Verification items for the finished model (mm, model axes). A direction names the side the tool comes from. Give positions to 0.01 mm unless a question says otherwise; leave off trailing zeros. Write each loop counter-clockwise with the first axis right and the second up, starting at its lowest first coordinate (ties: lowest second). Pieces come first, ordered by that corner, then holes. Notation, with made-up numbers: (83, -5) -> (89, -5) arc R26 ccw to (89, 14) -> close; hole circle Ø8 at (33.5, -25.5). An arc over 180 degrees is marked (long way). Use CSV: the item, a comma, the result in double quotes. Start each with the question number.
```python
from build123d import *

# Parameters (mm, degrees)
SKETCH1_R           = 1.5
BOSS_EXTRUDE1_DEPTH = 5
SKETCH2_R           = 6.375
CUT_EXTRUDE1_DEPTH  = 10
SKETCH3_W           = 16
SKETCH3_H           = 24.75
CUT_EXTRUDE2_DEPTH  = 10
FILLET1_R           = 2


with BuildPart() as part:
    # Sketch1 → Boss-Extrude1 (new body)
    with BuildSketch(Plane(origin=(0, 0, 0), x_dir=(1, 0, 0), z_dir=(0, 1, 0))):
        Polygon((5, -14), (19, -14), (19, -9), (24, -9), (24, 48.5), (19, 48.5), (19, 53.5), (5, 53.5), (5, 48.5), (0, 48.5), (0, -9), (5, -9), align=None)
        with Locations(Location((12, 51, 0), (0, 0, 270))):
            Circle(SKETCH1_R, mode=Mode.SUBTRACT)
        with Locations(Location((12, -11.5, 0), (0, 0, 90))):
            Circle(SKETCH1_R, mode=Mode.SUBTRACT)
    extrude(amount=BOSS_EXTRUDE1_DEPTH)

    # Sketch2 → Cut-Extrude1 (cut)
    with BuildSketch(Plane(origin=(0, 5, 0), x_dir=(1, 0, 0), z_dir=(0, 1, 0))):
        with Locations(Location((12, 29.26, 0), (0, 0, 270))):
            Circle(SKETCH2_R)
    extrude(amount=-CUT_EXTRUDE1_DEPTH, mode=Mode.SUBTRACT)

    # Sketch3 → Cut-Extrude2 (cut)
    with BuildSketch(Plane(origin=(0, 5, 0), x_dir=(1, 0, 0), z_dir=(0, 1, 0))):
        with Locations((12, 7.375)):
            Rectangle(SKETCH3_W, SKETCH3_H)
    extrude(amount=-CUT_EXTRUDE2_DEPTH, mode=Mode.SUBTRACT)

    # Fillet1
    fillet1_edges = [part.edges().sort_by_distance(p)[0] for p in [
        (20, 2.5, 5),
        (4, 2.5, 5),
        (4, 2.5, -19.75),
        (20, 2.5, -19.75),
    ]]
    fillet(fillet1_edges, radius=FILLET1_R)


solid = part.part
```
(1) Set-up check for faces 4 (the face through (2, 2, 9)), 5 (the face through (12, 3, 5)), 6 (the face through (19, 2, 12)): record each of +Z, -Z, +X, -X, +Y, -Y from which the full face is reachable in a straight line by a thin tool's end or side.
(2) Go/stop test with flat-tipped pins: pin 1 (2.5 mm diameter, centred on x = 1.5, y = 1.5, fed in from +Z); pin 2 (1.5 mm diameter, centred on x = 2.5, y = 3, fed in from -Z); pin 3 (1.5 mm diameter, centred on y = 3, z = 10.5, fed in from +X). Record where each tip stops, or that it passes through.
(3) Section check C-C on y = 2.75. Record the cut outline in (x, z) (3 decimals), then the cut area to 3 significant figures.
(4) Section check B-B on x = 12. Record the cut outline in (y, z) (3 decimals), then the cut area to 3 significant figures.
(5) Draft check along Z on faces 1 (the face through (3, 2, -48.5)), 2 (the face through (20, 3, -7)), 3 (the face through (12, 5, -20)). Enter one of: released by +Z, released by -Z, zero draft, split by the parting line, or undercut.
(6) Section check D-D on z = -29.26. Record the cut outline in (x, y) (3 decimals), then the cut area to 4 significant figures.
(7) Section check A-A on z = -51. Record the cut outline in (x, y), then the cut area to 3 significant figures.
(8) Thickness scan on line 1 (X direction, y = 1.3, z = 11.5); line 2 (Z direction, x = 6.75, y = 2.45); line 3 (Z direction, x = 9, y = 1.45) (3 decimals). Record the ranges inside material, lowest first. Write a range as from..to.
Data:
1,face 4,"+Z, -X, +Y, -Y"
1,face 5,"+Y, -Y"
1,face 6,"+Z, +X, +Y, -Y"
2,pin 1,"stops at z = 9"
2,pin 2,"stops at z = -48.5"
2,pin 3,"stops at x = 19"
3,outline,"(0, -48.5) -> (5, -48.5) -> (5, -53.5) -> (19, -53.5) -> (19, -48.5) -> (24, -48.5) -> (24, 9) -> (19, 9) -> (19, 14) -> (5, 14) -> (5, 9) -> (0, 9) -> close; hole (4, -17.75) arc R2 ccw to (6, -19.75) -> (18, -19.75) arc R2 ccw to (20, -17.75) -> (20, 3) arc R2 ccw to (18, 5) -> (6, 5) arc R2 ccw to (4, 3) -> close; hole circle Ø12.75 at (12, -29.26); hole circle Ø3 at (12, -51); hole circle Ø3 at (12, 11.5)"
3,area,"986 mm2"
4,outline,"(0, -53.5) -> (5, -53.5) -> (5, -52.5) -> (0, -52.5) -> close; (0, -49.5) -> (5, -49.5) -> (5, -35.635) -> (0, -35.635) -> close; (0, -22.885) -> (5, -22.885) -> (5, -19.75) -> (0, -19.75) -> close; (0, 5) -> (5, 5) -> (5, 10) -> (0, 10) -> close; (0, 13) -> (5, 13) -> (5, 14) -> (0, 14) -> close"
4,area,"120 mm2"
5,face 1,"released by -Z"
5,face 2,"undercut"
5,face 3,"zero draft"
6,outline,"(0, 0) -> (5.625, 0) -> (5.625, 5) -> (0, 5) -> close; (18.375, 0) -> (24, 0) -> (24, 5) -> (18.375, 5) -> close"
6,area,"56.25 mm2"
7,outline,"(5, 0) -> (10.5, 0) -> (10.5, 5) -> (5, 5) -> close; (13.5, 0) -> (19, 0) -> (19, 5) -> (13.5, 5) -> close"
7,area,"55.0 mm2"
8,line 1,"x = 5..10.5, 13.5..19"
8,line 2,"z = -53.5..-32.88, -25.64..-19.75, 5..14"
8,line 3,"z = -53.5..-34.885, -23.635..-19.75, 5..14"
